Autodesk Inventor part; units mm, degrees
ref_plane "YZ Plane" through (0, 0, 0) normal (1, 0, 0) x (0, 1, 0)
ref_plane "XZ Plane" through (0, 0, 0) normal (0, 1, 0) x (-1, 0, 0)
ref_plane "XY Plane" through (0, 0, 0) normal (0, 0, 1) x (1, 0, 0)
sketch "Skizze1" plane through (0, 0, 0) normal (0, 0, 1) x (1, 0, 0)
  line L0 (-15, 2) -> (-15, -2)
  line L1 (-15, -2) -> (15, -2)
  line L2 (15, -2) -> (15, 2)
  line L3 (15, 2) -> (-15, -2) construction
  line L4 (-15, 2) -> (15, -2) construction
  line L5 (-15, 2) -> (-6.65, 2) construction
  line L6 (15, 2) -> (6.65, 2) construction
  line L7 (-6.65, 2) -> (-6.65, 6)
  line L8 (-6.65, 6) -> (-5.387, 6)
  line L9 (6.65, 2) -> (6.65, 6)
  line L10 (6.65, 6) -> (5.387, 6)
  line L11 (-5.387, 6) -> (-2.248, 11.4369)
  line L12 (-5.387, 6) -> (0.891, 6) construction
  line L13 (5.387, 6) -> (2.248, 11.4369)
  line L14 (5.387, 6) -> (11.665, 6) construction
  arc A0 (2.248, 11.4369) -> (-2.248, 11.4369) centre (0, 16.9999) ccw
  line L15 (15, 2) -> (6.65, 2)
  line L16 (-6.65, 2) -> (-15, 2)
  point P0 (0, 0)
  dimension "d0" = 30
  dimension "d1" = 4
  dimension "d2" = 8.35
  dimension "d3" = 8.35
  dimension "d4" = 4
  dimension "d5" = 1.263
  dimension "d6" = 4
  dimension "d7" = 1.263
  dimension "d8" = 6.278
  dimension "d9" = 60
  dimension "d10" = 6.278
  dimension "d11" = 120
  dimension "d12" = 6
extrude "Extrusion1" add sketch "Skizze1" along normal blind 1000
properties part number "1000mmFührung" material "Edelstahl, 440C"
Work out the finished part from the listing and answer in its coordinate system (mm). Round coordinates to 2 decimals unless told otherwise and drop trailing zeros. Write each loop counter-clockwise with the first axis right and the second up, starting at its lowest first coordinate (ties: lowest second). Pieces come first, ordered by that corner, then holes. Notation, with made-up numbers: M -20,-36.75 L 19,-36.75 A16 cw 19,-15.75 Z; hole C 63,18.5 d3. An arc over 180 degrees is marked long. Use a Markdown table: item, result.
1) Consider line 1 (X direction, y = 18.5, z = 751); line 2 (X direction, y = 3, z = 319); line 3 (Y direction, x = 7.5, z = 388). Determine where each line is inside the solid, lowest interval first. Write a range as [from, to].
Taken from the geometry:
| item | result |
|---|---|
| line 1 | x = [-5.81, 5.81] |
| line 2 | x = [-6.65, 6.65] |
| line 3 | y = [-2, 2] |
2) Flat-ended cylindrical pins translate along their axes: pin 1 (1 mm diameter, centred on y = 9.5, z = 201, fed in from -X); pin 2 (0.6 mm diameter, centred on x = -6.5, z = 624.5, fed in from +Y); pin 3 (3 mm diameter, centred on y = 10.5, z = 310, fed in from +X). Find the tip coordinate at first contact, or state that the pin passes through.
Taken from the geometry:
| item | result |
|---|---|
| pin 1 | stops at x = -3.65 |
| pin 2 | stops at y = 6 |
| pin 3 | stops at x = 3.65 |
3) The part is cut by section A-A on z = 471. Give the vertices of the cut face in (x, y), plus the area to 3 significant figures.
Taken from the geometry:
| item | result |
|---|---|
| outline | M -15,-2 L 15,-2 L 15,2 L 6.65,2 L 6.65,6 L 5.39,6 L 2.25,11.44 A6 ccw long -2.25,11.44 L -5.39,6 L -6.65,6 L -6.65,2 L -15,2 Z |
| area | 326 mm2 |
